Geometry: see drawing. Coordinates: mm, zero at the bounding-box minimum. Coordinates: 2 decimals unless noted, no trailing zeros. Order: outer loops, then holes, each group sorted by start corner. A loop starts at its lowest first (then second) coordinate and runs counter-clockwise, first axis right, second up. Notation, with made-up numbers: (37, 80.5) - (45, 80.5) arc R26 cw to (45, 113.5) - close; hole circle Ø3 at (30, 64). An arc over 180 degrees is marked (long way). Use a Markdown table: item, result. Add a question column.
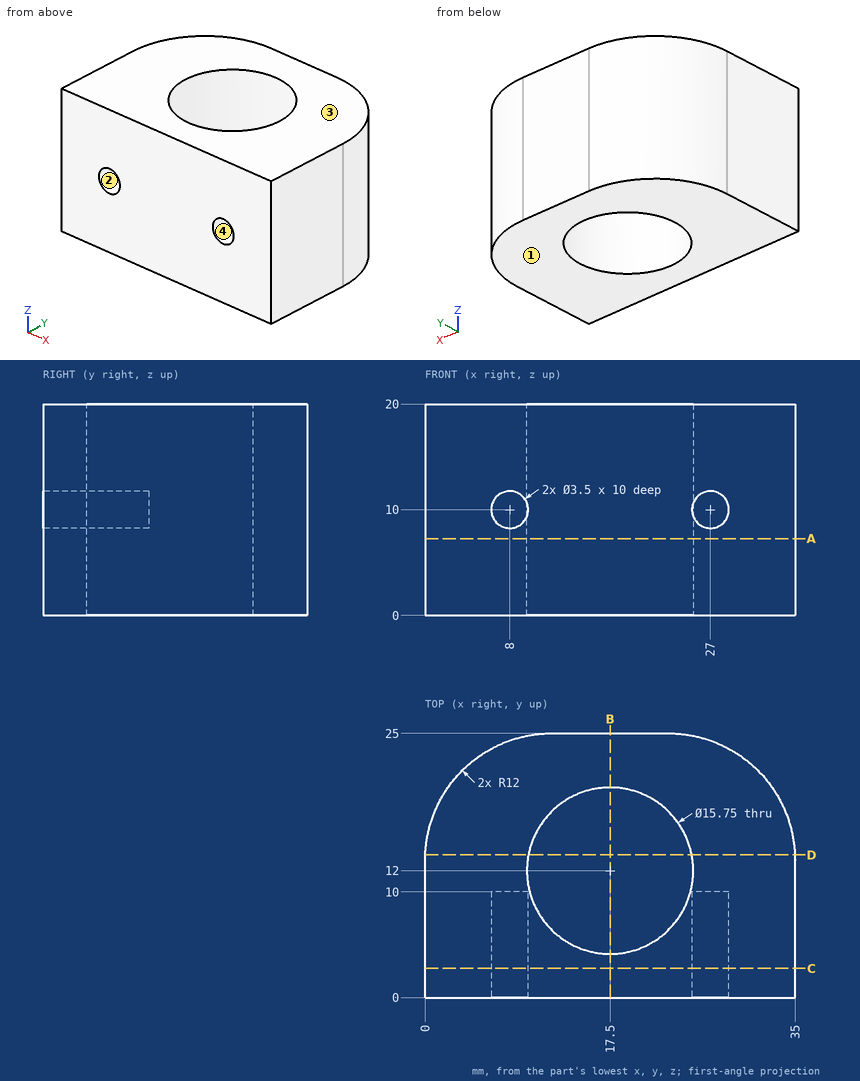
1) Section query A-A (z = 7.25). Return the cut outline in (x, y) (3 decimals).
2) Section query B-B (x = 17.5). Return the cut outline in (y, z) (3 decimals).
3) Section query C-C (y = 2.75). Return the cut outline in (x, z), and give its area (3 significant figures).
4) First-contact query: pin 1 (4.5 mm diameter, centred on x = 27, z = 10, fed in from +Y); pin 2 (3 mm diameter, centred on x = 8, z = 10, fed in from -Y); pin 3 (2 mm diameter, centred on y = 20, z = 10.5, fed in from -X). Flat tips, straight axial feed; report the tip coordinate or a pass-through.
5) Section query D-D (y = 13.5). Return the cut outline in (x, z).
6) Line query: line 1 (Z direction, x = 8, y = 5.75); line 2 (Y direction, x = 17.5, z = 11.25) (3 decimals); line 3 (X direction, y = 2.5, z = 9). Output: solid intervals per line, ascending. Write a range as from..to.
7) Draft query along Z for the marked faces 1, 2, 3 and 4. Return one class per face: released by +Z, released by -Z, zero draft, split by the parting line, or undercut.
From the geometry:
| question | item | result |
|---|---|---|
| 1 | outline | (0, 0) - (35, 0) - (35, 13) arc R12 ccw to (23, 25) - (12, 25) arc R12 ccw to (0, 13) - close; hole circle Ø15.75 at (17.5, 12) |
| 2 | outline | (0, 0) - (4.125, 0) - (4.125, 20) - (0, 20) - close; (19.875, 0) - (25, 0) - (25, 20) - (19.875, 20) - close |
| 3 | outline | (0, 0) - (35, 0) - (35, 20) - (0, 20) - close; hole circle Ø3.5 at (8, 10); hole circle Ø3.5 at (27, 10) |
| 3 | area | 681 mm^2 |
| 4 | pin 1 | stops at y = 24.87 |
| 4 | pin 2 | stops at y = 10 |
| 4 | pin 3 | stops at x = 1.61 |
| 5 | outline | (0.01, 0) - (9.77, 0) - (9.77, 20) - (0.01, 20) - close; (25.23, 0) - (34.99, 0) - (34.99, 20) - (25.23, 20) - close |
| 6 | line 1 | z = 0..8.25, 11.75..20 |
| 6 | line 2 | y = 0..4.125, 19.875..25 |
| 6 | line 3 | x = 0..6.56, 9.44..25.56, 28.44..35 |
| 7 | face 1 | released by -Z |
| 7 | face 2 | undercut |
| 7 | face 3 | released by +Z |
| 7 | face 4 | undercut |
